Could you check a few things on this model? Use its own coordinates, in mm. A direction names the side the tool comes from. Coordinates: 2 decimals unless noted, no trailing zeros. Write each loop counter-clockwise with the first axis right and the second up, starting at its lowest first coordinate (ties: lowest second). Pieces come first, ordered by that corner, then holes.
```python
from build123d import *

# Parameters (mm, degrees)
F1_DEPTH = 0.6096
F2_R     = 0.381
F3_DEPTH = 25.4
F4_R     = 0.127
F5_DEPTH = 2.54
F6_R     = 0.6858
F6_R_2   = 0.381
F7_DEPTH = 0.508


with BuildPart() as f1:
    # F0 (on Top) → F1 (new body)
    with BuildSketch(Plane.XY):
        Polygon((1.27, 0.762), (-1.27, 0.762), (-3.81, 0.4572), (-5.842, 0.4572), (-5.842, -0.4572), (-3.81, -0.4572), (-2.998233, -0.554612), (-2.296821, -0.638781), (-1.27, -0.762), (1.27, -0.762), (3.81, -0.4572), (5.842, -0.4572), (5.842, 0.4572), (3.81, 0.4572), align=None)
        Polygon((-2.296821, -0.638781), (-2.998233, -0.554612), (-3.471884, -1.405351), (-2.900672, -1.723375), align=None)
    extrude(amount=F1_DEPTH)

    # F2 (on face) → F3 (cut)
    with BuildSketch(Plane.XY.offset(0.6096)):
        Circle(F2_R)
    extrude(amount=-F3_DEPTH, mode=Mode.SUBTRACT)

    # F4 (on face) → F5 (cut)
    with BuildSketch(Plane.XY.offset(0.6096)):
        with Locations((-5.334, 0)):
            Circle(F4_R)
        with Locations((5.334, 0)):
            Circle(F4_R)
    extrude(amount=-F5_DEPTH, mode=Mode.SUBTRACT)

    # F6 (on Top) → F7 (join)
    with BuildSketch(Plane.XY):
        Circle(F6_R)
        Circle(F6_R_2, mode=Mode.SUBTRACT)
    extrude(amount=-F7_DEPTH)


solid = f1.part
```
1. I want a section at A-A on x = 0. Please give me the cut outline in (y, z).
Verdict:
outline: (-0.76, 0) - (-0.69, 0) - (-0.69, -0.51) - (-0.38, -0.51) - (-0.38, 0.61) - (-0.76, 0.61) - close; (0.38, -0.51) - (0.69, -0.51) - (0.69, 0) - (0.76, 0) - (0.76, 0.61) - (0.38, 0.61) - close
2. I want a section at B-B on y = 0. Please give me the cut outline in (x, z), plus the area to 3 significant figures.
Verdict:
outline: (-5.84, 0) - (-5.46, 0) - (-5.46, 0.61) - (-5.84, 0.61) - close; (-5.21, 0) - (-0.69, 0) - (-0.69, -0.51) - (-0.38, -0.51) - (-0.38, 0.61) - (-5.21, 0.61) - close; (0.38, -0.51) - (0.69, -0.51) - (0.69, 0) - (5.21, 0) - (5.21, 0.61) - (0.38, 0.61) - close; (5.46, 0) - (5.84, 0) - (5.84, 0.61) - (5.46, 0.61) - close
area: 6.66 mm2
3. For pin 1 (1 mm diameter, centred on x = 3, y = -0.5, fed in from -Z), with a flat end and sliding along its axis, tell me the tip position at first contact or that it passes through.
Verdict:
pin 1: stops at z = 0
4. I want a section at C-C on x = 1.75. Please give me the cut outline in (y, z).
Verdict:
outline: (-0.7, 0) - (0.7, 0) - (0.7, 0.61) - (-0.7, 0.61) - close
5. On a 3-axis mill with a long thin cutter (end or side, diameter ignored), from which of +Z, -Z, +X, -X, +Y, -Y can I reach the whole of each face in a straight line? I mean faces 1 (the face through (-0.15, -0.67, -0.25)), 2 (the face through (-0.1, 0.6, 0.61)). Say none if no direction works.
Verdict:
face 1: -Z
face 2: +Z, +X, -X, +Y, -Y
6. Please list where these lines run through material, in increasing order: line 1 along Y through (x, z) = (0, -0.2); line 2 along Y through (x, z) = (0, 0.05); line 3 along Z through (x, y) = (-1.25, 0.55).
Verdict:
line 1: y = -0.69 to -0.38, 0.38 to 0.69
line 2: y = -0.76 to -0.38, 0.38 to 0.76
line 3: z = 0 to 0.61
